Check sheet for the modelled part. Datum: model origin and axes. Units: mm. Give positions to 0.01 mm unless a question says otherwise; leave off trailing zeros. Order: outer loops, then holes, each group sorted by start corner. A loop starts at its lowest first (then second) coordinate and runs counter-clockwise, first axis right, second up. Notation, with made-up numbers: (-7, 3) - (36, 3) arc R21 cw to (36, 13) - close; hole circle Ø3 at (74, 35.25). An arc over 180 degrees is marked (long way). Answer in a Markdown table with one row per item.
Autodesk Inventor part; units mm, degrees
ref_plane "YZ Plane" through (0, 0, 0) normal (1, 0, 0) x (0, 1, 0)
ref_plane "XZ Plane" through (0, 0, 0) normal (0, 1, 0) x (-1, 0, 0)
ref_plane "XY Plane" through (0, 0, 0) normal (0, 0, 1) x (1, 0, 0)
sketch "Sketch2" plane through (0, 0, 0) normal (0, 0, 1) x (1, 0, 0)
  line L0 (4.8719, 5.1626) -> (-7.644, -2.8311)
  line L1 (5.3481, 4.5174) -> (-5.1907, -2.2135)
  line L2 (5.3481, 4.5174) -> (6.0672, 4.9767)
  arc A0 (-5.1907, -2.2135) -> (-7.644, -2.8311) centre (-5.4909, -6.2022) ccw
  line L3 (6.0672, 4.9767) -> (4.8719, 5.1626)
  point P0 (5.2456, 5.1046)
  dimension "d8" = 0.8
  dimension "d9" = 8
extrude "Extrusion2" add sketch "Sketch2" along normal blind 142
properties part number "2P.03.01.06.IM.AileronCutFill" material "Wood (Birch)"
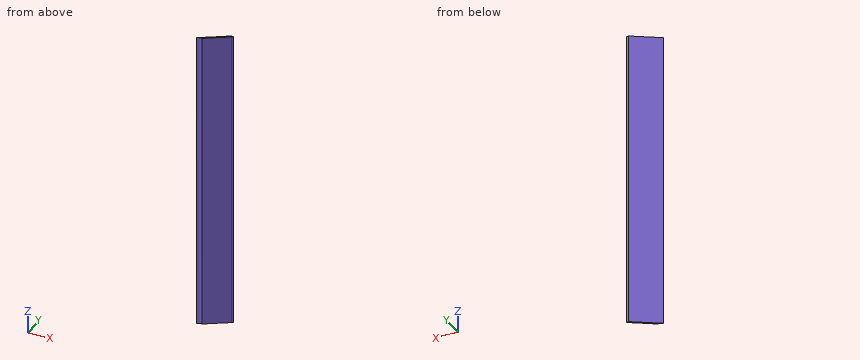
(1) Cross-section at C-C, the plane y = 2. Record the cut outline in (x, z), then the cut area to 3 significant figures.
Geometry says:
| item | result |
|---|---|
| outline | (-0.08, 0) - (1.41, 0) - (1.41, 142) - (-0.08, 142) - close |
| area | 211 mm² |
(2) Gauge pin test, flat ends, axial feed: P1, Ø3, axis at x = -4, z = 47.5, coming from the +Y side; P2, Ø3, axis at y = 3.5, z = 72.5, coming from the -X side; P3, Ø5, axis at x = -3, z = 122.5, coming from the -Y side. Record the tip position at first contact, or that the pin passes through.
Geometry says:
| item | result |
|---|---|
| P1 | y = 0.45 |
| P2 | x = -0.08 |
| P3 | y = -2.21 |
(3) Thickness scan on L1, parallel to Y at x = -5, z = 39.5; L2, parallel to X at y = 1.5, z = 50; L3, parallel to X at y = -1.75, z = 30. Record the ranges inside material, lowest first.
Geometry says:
| item | result |
|---|---|
| L1 | -2.09 to -1.14 |
| L2 | -0.86 to 0.62 |
| L3 | -5.95 to -4.46 |
(4) Cross-section at A-A, the plane z = 131. Record the cut outline in (x, y), then the cut area to 3 significant figures.
Geometry says:
| item | result |
|---|---|
| outline | (-7.64, -2.83) arc R4 cw to (-5.19, -2.21) - (5.35, 4.52) - (6.07, 4.98) - (4.87, 5.16) - close |
| area | 10.9 mm² |
(5) Cross-section at B-B, the plane x = 2.25. Record the cut outline in (y, z), then the cut area to 3 significant figures.
Geometry says:
| item | result |
|---|---|
| outline | (2.54, 0) - (3.49, 0) - (3.49, 142) - (2.54, 142) - close |
| area | 135 mm² |
